Check sheet for the modelled part. Datum: model origin and axes. Units: mm. A direction names the side the tool comes from. Round coordinates to 2 decimals unless told otherwise and drop trailing zeros. Write each loop counter-clockwise with the first axis right and the second up, starting at its lowest first coordinate (ties: lowest second). Pieces come first, ordered by that corner, then holes. Notation, with made-up numbers: (75.25, -38.5) - (104.25, -38.5) arc R9 ccw to (104.25, -27.5) - close; hole circle Ø1 at (-0.75, -35.75). An arc over 180 degrees is marked (long way). Answer as a JSON object with one key per item and string values. Group by question number.
Item 1: Gauge pin test, flat ends, axial feed: P1, Ø1.5, axis at x = 2, y = 10, coming from the +Z side (3 decimals); P2, Ø1, axis at x = -10.5, z = 9.5, coming from the +Y side; P3, Ø5.5, axis at x = 9.525, z = 9.525, coming from the +Y side (3 decimals). Record the tip position at first contact, or that the pin passes through.
Item 2: Sectioned sample at D-D on z = 9. Record the boundary of the cut face in (x, y) (3 decimals), plus the area to 3 significant figures.
Item 3: Set-up check for faces 1 (the flat face through (0, -6, 3.175)), 2 (the cylindrical face through (5.3, 1.67, 1.61)): record each of +Z, -Z, +X, -X, +Y, -Y from which the full face is reachable in a straight line by a thin tool's end or side.
Item 4: Release check for a two-part mould opening along Y. For faces 3 (the cylindrical face through (-7, 0, 2)), 4 (the cylindrical face through (0.35, 15.87, 1.57)), 5 (the cylindrical face through (8.8, -0.6, 2)), 6 (the flat face through (0, -8, 0)) record: pulls with the +Y half, pulls with the -Y half, needs draft (parallel to the pull), parting line crosses it, or undercut.
Item 5: Sectioned sample at A-A on x = 0. Record the boundary of the cut face in (y, z) (3 decimals), plus the area to 3 significant figures.
Item 6: Sectioned sample at B-B on z = 1.5. Count the separate pieces of the cut face and the enclosed holes in it, plus the area to 3 significant figures.
Item 7: Sectioned sample at C-C on y = -16.5. Record the boundary of the cut face in (x, z) (3 decimals).
Item 8: Thickness scan on line 1 (Y direction, x = 0, z = 2.05) (3 decimals); line 2 (Y direction, x = 2.5, z = 10.75) (3 decimals); line 3 (Z direction, x = -12, y = -17.5) (3 decimals). Record the ranges inside material, lowest first.
```python
from build123d import *

# Parameters (mm, degrees)
BOSS_EXTRUDE1_DEPTH       = 3.175
SKETCH3_R                 = 5.55625
CUT_EXTRUDE1_DEPTH        = 36.639286609
SKETCH4_W                 = 31.75
SKETCH4_H                 = 3.175
BOSS_EXTRUDE2_DEPTH       = 12.7
SKETCH5_R                 = 1.75
CUT_EXTRUDE2_DEPTH        = 50.797929174
F_2_0MM_DOWEL_HOLE1_D     = 2
F_2_0MM_DOWEL_HOLE1_DEPTH = 12.7
F_2_0MM_DOWEL_HOLE1_TIP   = 0.600860619
CHAMFER1_SIZE             = 0.762


with BuildPart() as part:
    # Sketch1 → Boss-Extrude1 (new body)
    with BuildSketch(Plane.XY):
        with BuildLine():
            ThreePointArc((15.875, 0), (0, 15.875), (-15.875, 0))
            Line((-15.875, 0), (15.875, 0))
        make_face()
        with BuildLine():
            ThreePointArc((15.875, 0), (0, -15.875), (-15.875, 0))
            Line((-15.875, 0), (-15.875, -31.75))
            Line((-15.875, -31.75), (15.875, -31.75))
            Line((15.875, -31.75), (15.875, 0))
        make_face()
        with BuildLine():
            Line((15.875, 0), (-15.875, 0))
            ThreePointArc((-15.875, 0), (0, -15.875), (15.875, 0))
        make_face()
    extrude(amount=BOSS_EXTRUDE1_DEPTH)

    # Sketch3 → Cut-Extrude1 (cut, through all)
    with BuildSketch(Plane.XY.offset(3.175)):
        Circle(SKETCH3_R)
    extrude(amount=-CUT_EXTRUDE1_DEPTH, mode=Mode.SUBTRACT)

    # Sketch4 → Boss-Extrude2 (add)
    with BuildSketch(Plane.XY.offset(3.175)):
        with Locations((0, -30.1625)):
            Rectangle(SKETCH4_W, SKETCH4_H)
    extrude(amount=BOSS_EXTRUDE2_DEPTH)

    # Sketch5 → Cut-Extrude2 (cut, through all)
    with BuildSketch(Plane(origin=(0, -28.575, 0), x_dir=(1, 0, 0), z_dir=(0, 1, 0))):
        with Locations(Location((-9.525, -9.525, 0), (0, 0, 270))):
            Circle(SKETCH5_R)
        with Locations(Location((9.525, -9.525, 0), (0, 0, 90))):
            Circle(SKETCH5_R)
    extrude(amount=-CUT_EXTRUDE2_DEPTH, mode=Mode.SUBTRACT)

    # Ø2.0mm Dowel Hole1
    with Locations(Plane.XY.offset(3.175)):
        with Locations((-8.001, 0), (8.001, 0)):
            Hole(F_2_0MM_DOWEL_HOLE1_D / 2, depth=F_2_0MM_DOWEL_HOLE1_DEPTH)
            with Locations((0, 0, -(F_2_0MM_DOWEL_HOLE1_DEPTH + F_2_0MM_DOWEL_HOLE1_TIP / 2))):  # 118° drill point
                Cone(0, F_2_0MM_DOWEL_HOLE1_D / 2, F_2_0MM_DOWEL_HOLE1_TIP, mode=Mode.SUBTRACT)

    # Chamfer1
    chamfer1_edges = [part.edges().sort_by_distance(p)[0] for p in [
        (9.001, 0, 0),
        (-7.001, 0, 0),
    ]]
    chamfer(chamfer1_edges, length=CHAMFER1_SIZE)


solid = part.part
```
Completed:
{
 "1": {"P1": "z = 3.175", "P2": "through", "P3": "y = -28.575"},
 "2": {"outline": "(-15.875, -31.75) - (-11.194, -31.75) - (-11.194, -28.575) - (-15.875, -28.575) - close; (-7.856, -31.75) - (7.856, -31.75) - (7.856, -28.575) - (-7.856, -28.575) - close; (11.194, -31.75) - (15.875, -31.75) - (15.875, -28.575) - (11.194, -28.575) - close", "area": "79.6 mm²"},
 "3": {"face 1": "+Z, +X, -X, +Y", "face 2": "+Z, -Z"},
 "4": {"face 3": "undercut", "face 4": "pulls with the +Y half", "face 5": "undercut", "face 6": "needs draft"},
 "5": {"outline": "(-31.75, 0) - (-5.556, 0) - (-5.556, 3.175) - (-28.575, 3.175) - (-28.575, 15.875) - (-31.75, 15.875) - close; (5.556, 0) - (15.875, 0) - (15.875, 3.175) - (5.556, 3.175) - close", "area": "156 mm²"},
 "6": {"separate pieces": "1", "enclosed holes": "3", "area": "1,300 mm²"},
 "7": {"outline": "(-15.875, 0) - (15.875, 0) - (15.875, 3.175) - (-15.875, 3.175) - close"},
 "8": {"line 1": "-31.75 to -5.556, 5.556 to 15.875", "line 2": "-31.75 to -28.575", "line 3": "0 to 3.175"}
}
